from build123d import *

# Parameters (mm, degrees)
SKETCH_R             = 5.95
PAD_DEPTH            = 3.5
POCKET_DEPTH         = 3.5
POLARPATTERN_COUNT   = 20
SKETCH002_R          = 7.5
PAD001_DEPTH         = 3
SKETCH003_R          = 7.5
PAD002_DEPTH         = 5
FILLET_R             = 1
SKETCH005_R          = 2.5
POCKET002_DEPTH      = 6.501
POCKET002_DEPTH_BACK = -8.501


with BuildPart() as part:
    # Sketch → Pad (new body, symmetric)
    with BuildSketch(Plane.XY):
        Circle(SKETCH_R)
    extrude(amount=PAD_DEPTH, both=True)

    # Sketch001 → Pocket (cut, symmetric)
    with BuildSketch(Plane.XY):
        with BuildLine():
            ThreePointArc((-0.495406, 5.477643), (-0.697454, 5.814914), (-1.080885, 5.901838))
            ThreePointArc((1.080885, 5.901838), (0, 6), (-1.080885, 5.901838))
            ThreePointArc((1.080885, 5.901838), (0.697454, 5.814914), (0.495406, 5.477643))
            ThreePointArc((-0.495406, 5.477643), (0, 5.045268), (0.495406, 5.477643))
        make_face()
    pocket = extrude(amount=POCKET_DEPTH, both=True, mode=Mode.SUBTRACT)

    # PolarPattern: Pocket ×20 about axis
    polarpattern_axis = Axis((0, 0, 0), (0, 0, 1))
    for i in range(1, POLARPATTERN_COUNT):
        add(pocket.rotate(polarpattern_axis, i * 360 / POLARPATTERN_COUNT), mode=Mode.SUBTRACT)

    # Sketch002 (on Face2 of PolarPattern) → Pad001 (join)
    with BuildSketch(Plane(origin=(0, 0, -3.5), x_dir=(1, 0, 0), z_dir=(0, 0, -1))):
        Circle(SKETCH002_R)
    extrude(amount=PAD001_DEPTH)

    # Sketch003 → Pad002 (join)
    with BuildSketch(Plane.XY.offset(3.5)):
        Circle(SKETCH003_R)
    extrude(amount=PAD002_DEPTH)

    # Fillet
    fillet_edges = [part.edges().sort_by_distance(p)[0] for p in [
        (7.5, 0, 6),
        (-7.5, 0, 3.5),
        (-7.5, 0, 8.5),
        (7.5, 0, -5),
        (-7.5, 0, -3.5),
        (-7.5, 0, -6.5),
    ]]
    fillet(fillet_edges, radius=FILLET_R)

    # Sketch005 → Pocket002 (cut, two sides)
    with BuildSketch(Plane.XY) as pocket002_sk:
        Circle(SKETCH005_R)
    extrude(amount=-POCKET002_DEPTH, mode=Mode.SUBTRACT)
    extrude(pocket002_sk.sketch, amount=-POCKET002_DEPTH_BACK, mode=Mode.SUBTRACT)


solid = part.part
CAD build for the part. Positions are in the model's coordinates, mm. A direction names the side the tool comes from. Round coordinates to 2 decimals unless told otherwise and drop trailing zeros. Loops run counter-clockwise (first coordinate to the right, second up) from the corner with the lowest first, then second, coordinate; pieces in that order, holes last.
(1) Drop flat-ended pins along their axis: pin 1 (3 mm diameter, centred on x = 0, y = 0, fed in from -Z); pin 2 (6 mm diameter, centred on x = -4.5, z = -4.5, fed in from +Y); pin 3 (6 mm diameter, centred on y = 5.5, z = 3.5, fed in from -X); pin 4 (3 mm diameter, centred on x = -3, z = 0, fed in from +Y). Give the stop position or say it passes through.
(2) Cut at A-A (x = 0). Give the cut face in (y, z), plus the area to 3 significant figures.
(3) Which spindle directions (+Z, -Z, +X, -X, +Y, -Y) get a long thin tool onto all of the face, cutting with end or side? Do faces 4 (the flat face through (0, -5.3, 3.5)), 5 (the flat face through (3, 0, 8.5)). Say none if no direction does.
(4) Two-plate mould, pull along Z, no slides. Class faces 1 (the flat face through (3, 0, -6.5)), 2 (the cylindrical face through (-7.493, -0.33, -4.993)), 3 (the flat face through (0, 5.3, -3.5)): +Z half, -Z half, draft (parallel to the pull), parting line (faces both ways), or undercut.
(5) Wall check: line 1 along Z through (x, y) = (-5.5, -2.5); line 2 along Y through (x, z) = (0, -4.5); line 3 along X through (y, z) = (5.5, -0.75). Give the ranges that are in metal, low to high.
Findings below:
1. pin 1: passes through
1. pin 2: stops at y = 7.35
1. pin 3: stops at x = -7.02
1. pin 4: stops at y = 5.34
2. outline: (-7.5, -5.5) arc R1 ccw to (-6.5, -6.5) - (-2.5, -6.5) - (-2.5, 8.5) - (-6.5, 8.5) arc R1 ccw to (-7.5, 7.5) - (-7.5, 4.5) arc R1 ccw to (-6.5, 3.5) - (-5.05, 3.5) - (-5.05, -3.5) - (-6.5, -3.5) arc R1 ccw to (-7.5, -4.5) - close; (2.5, -6.5) - (6.5, -6.5) arc R1 ccw to (7.5, -5.5) - (7.5, -4.5) arc R1 ccw to (6.5, -3.5) - (5.05, -3.5) - (5.05, 3.5) - (6.5, 3.5) arc R1 ccw to (7.5, 4.5) - (7.5, 7.5) arc R1 ccw to (6.5, 8.5) - (2.5, 8.5) - close
2. area: 114 mm2
3. face 4: none
3. face 5: +Z, +X, -X, +Y, -Y
4. face 1: -Z half
4. face 2: draft
4. face 3: undercut
5. line 1: z = -6.5 to -3.5, 3.5 to 8.5
5. line 2: y = -7.5 to -2.5, 2.5 to 7.5
5. line 3: x = -1.23 to -0.5, 0.5 to 1.23
